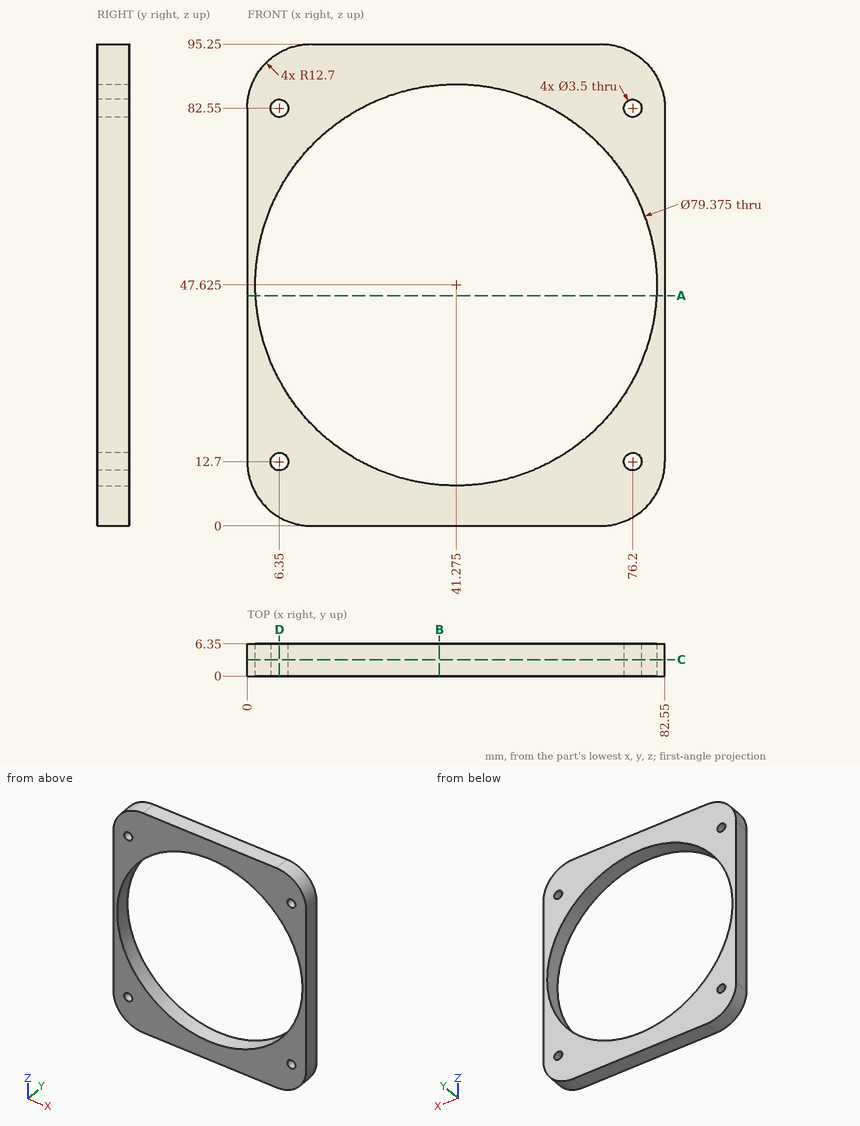
Here's the drawing with two shaded views (mm, measured from the low corner). I have some questions. Give positions to 0.01 mm unless a question says otherwise; leave off trailing zeros. Loops run counter-clockwise (first coordinate to the right, second up) from the corner with the lowest first, then second, coordinate; pieces in that order, holes last. Notation, with made-up numbers: M -39.75,-28.5 L -28.75,-28.5 A19 ccw -28.75,-23.5 Z; hole C 8.25,-5 d8. An arc over 180 degrees is marked long. One line per item, written item: value.
1) Imagine slicing it at B-B on x = 38. Write out the boundary of the cut face in (y, z).
Geometry check:
outline: M 0,0 L 6.35,0 L 6.35,8.07 L 0,8.07 Z; M 0,87.18 L 6.35,87.18 L 6.35,95.25 L 0,95.25 Z
2) Imagine slicing it at C-C on y = 3.25. Count the separate pieces of the cut face and the enclosed holes in it, and give its area (3 significant figures).
Geometry check:
separate pieces: 1
enclosed holes: 5
area: 2,740 mm²
3) Please list where these lines run through material, in increasing order: line 1 (Z direction, x = 76.2, y = 3.5); line 2 (X direction, y = 1.75, z = 11.5); line 3 (X direction, y = 4.5, z = 13).
Geometry check:
line 1: z = 1.7 to 10.95, 14.45 to 28.77, 66.48 to 80.8, 84.3 to 93.55
line 2: x = 0.06 to 5.08, 7.62 to 24.84, 57.71 to 74.93, 77.47 to 82.49
line 3: x = 0 to 4.63, 8.07 to 21.88, 60.67 to 74.48, 77.92 to 82.55
4) I'm going to push a flat-ended pin straight in: pin 1 (2 mm diameter, centred on x = 76.2, z = 12.7, fed in from +Y). Where does the tip first touch, or does it pass through?
Geometry check:
pin 1: passes through
5) Imagine slicing it at D-D on x = 6.35. Write out the boundary of the cut face in (y, z).
Geometry check:
outline: M 0,1.7 L 6.35,1.7 L 6.35,10.95 L 0,10.95 Z; M 0,14.45 L 6.35,14.45 L 6.35,28.77 L 0,28.77 Z; M 0,66.48 L 6.35,66.48 L 6.35,80.8 L 0,80.8 Z; M 0,84.3 L 6.35,84.3 L 6.35,93.55 L 0,93.55 Z
6) Imagine slicing it at A-A on z = 45.5. Write out the boundary of the cut face in (x, y), and give its area (3 significant figures).
Geometry check:
outline: M 0,0 L 1.64,0 L 1.64,6.35 L 0,6.35 Z; M 80.91,0 L 82.55,0 L 82.55,6.35 L 80.91,6.35 Z
area: 20.9 mm²
